```python
from build123d import *

# Parameters (mm, degrees)
SKETCH1_R           = 3.6
BOSS_EXTRUDE1_DEPTH = 4
FILLET1_DEPTH       = 4


with BuildPart() as part:
    # Sketch1 → Boss-Extrude1 (new body)
    with BuildSketch(Plane(origin=(0, 0, 0), x_dir=(1, 0, 0), z_dir=(0, 1, 0))):
        with BuildLine():
            Line((9.346086984, -56.356572977), (15.081851343, -64.548093422))
            ThreePointArc((15.081851343, -64.548093422), (27.699790534, -36.740032424), (9.415453774, -12.282238674))
            ThreePointArc((9.415453774, -12.282238674), (6.074212989, -8.697213495), (6.569252548, -3.821638518))
            ThreePointArc((6.569252548, -3.821638518), (1.956261977, 7.343911701), (-7.599852871, -0.04729001))
            ThreePointArc((-7.599852871, -0.04729001), (-3.773263774, -12.975309302), (6.3636811, -21.864562113))
            ThreePointArc((6.3636811, -21.864562113), (17.800210223, -38.250629299), (9.346086984, -56.356572977))
        make_face()
        with Locations(Location((0, 0, 0), (0, 0, 270))):
            Circle(SKETCH1_R, mode=Mode.SUBTRACT)
    extrude(amount=BOSS_EXTRUDE1_DEPTH)

    # Fillet1: read off the stored shape, not the designer's step
    # Fillet1 outline → Fillet1 (cut)
    with BuildSketch(Plane(origin=(0, 0, 0), x_dir=(1, 0, 0), z_dir=(0, 1, 0))):
        with BuildLine():
            ThreePointArc((15.081851343, -64.548093422), (17.464679897, -62.694164436), (19.649105693, -60.610127838))
            add(Edge.make_bspline(
                [(19.649105693, -60.610127838), (18.677855173, -61.634935456), (17.188222286, -62.496348841), (15.223722909, -62.743763995), (13.23213393, -61.906423138), (11.924254263, -60.03857744)],
                knots=[0, 0, 0, 0, 0, 0, 0.550510254, 0.550510254, 0.550510254, 0.550510254, 0.550510254, 0.550510254], degree=5, weights=[1, 0.779795898, 0.620204104, 0.521224619, 0.482857441, 0.505102571]))
            Line((11.924254263, -60.03857744), (15.081851343, -64.548093422))
        make_face()
        with BuildLine():
            Line((9.346086984, -56.356572977), (11.924254263, -60.03857744))
            add(Edge.make_bspline(
                [(11.924254263, -60.03857744), (10.93883994, -58.631259971), (10.675135711, -57.05607025), (10.993827945, -55.636809597), (11.636969564, -54.526791063), (12.390923216, -53.731262588)],
                knots=[0.550510254, 0.550510254, 0.550510254, 0.550510254, 0.550510254, 0.550510254, 1, 1, 1, 1, 1, 1], degree=5, weights=[0.505102571, 0.523265645, 0.581836924, 0.68081641, 0.820204102, 1]))
            ThreePointArc((12.390923216, -53.731262588), (10.934639353, -55.12062032), (9.346086984, -56.356572977))
        make_face()
    extrude(amount=FILLET1_DEPTH, mode=Mode.SUBTRACT)


solid = part.part
```
CAD build for the part. Positions are in the model's coordinates, mm. Give positions to 0.01 mm unless a question says otherwise; leave off trailing zeros. Write each loop counter-clockwise with the first axis right and the second up, starting at its lowest first coordinate (ties: lowest second). Pieces come first, ordered by that corner, then holes. Notation, with made-up numbers: M 71,89.25 L 76,89.25 A27 cw 76,122.25 Z; hole C 21.5,89 d5. An arc over 180 degrees is marked long. Return JSON: item names as keys, results as strings. Group by question number.
(1) Band-saw the part on B-B (z = 11). Give the cut face in (x, y), and give its area (3 significant figures).
(2) Drill centre lines: L1, parallel to X at y = 1.65, z = 0; L2, parallel to X at y = 2.6, z = -1.5; L3, parallel to Z at x = -3, y = 1.75. Where is each one in solid material? Low to high. Write a range as [from, to].
(3) Flat gauge pins, fed straight in: pin 1 Ø1 at (x, y) = (2.5, 0.5) entering from -Z; pin 2 Ø1.5 at (y, z) = (1.5, 36) entering from +X; pin 3 Ø1.5 at (y, z) = (1, 4.5) entering from +X. Where does each tip first touch, or does it go through?
(4) Mould opens along X. For faces 1 (the face through (14, 4, 27)), 2 (the face through (-1.379, 1.972, 3.325)), 3 (the face through (17.475, 1.972, 35.997)) say: pulls with the +X half, pulls with the -X half, needs draft (parallel to the pull), parting line crosses it, or undercut.
(5) Band-saw the part on A-A (x = 0). Give the cut face in (y, z), and give its area (3 significant figures).
(6) Band-saw the part on C-C (x = 26). Give the cut face in (y, z).
Entries:
{
 "1": {"outline": "M -4.91,0 L 7.5,0 L 7.5,4 L -4.91,4 Z", "area": "49.6 mm^2"},
 "2": {"L1": "x = [-7.6, -3.6], [3.6, 7.6]", "L2": "x = [-7.45, -3.27], [3.27, 7.45]", "L3": "z = [-6.98, -1.99], [1.99, 14.11]"},
 "3": {"pin 1": "stops at z = -7.33", "pin 2": "stops at x = 27.7", "pin 3": "stops at x = 6.61"},
 "4": {"face 1": "needs draft", "face 2": "undercut", "face 3": "pulls with the -X half"},
 "5": {"outline": "M 0,-7.6 L 4,-7.6 L 4,-3.6 L 0,-3.6 Z; M 0,3.6 L 4,3.6 L 4,17.53 L 0,17.53 Z", "area": "71.7 mm^2"},
 "6": {"outline": "M 0,29.54 L 4,29.54 L 4,50.41 L 0,50.41 Z"}
}
